Could you check a few things on this model? Use its own coordinates, in mm. Coordinates: 2 decimals unless noted, no trailing zeros. Write each loop counter-clockwise with the first axis right and the second up, starting at its lowest first coordinate (ties: lowest second). Pieces come first, ordered by that corner, then holes. Notation, with made-up numbers: M 69.5,-13 L 86.5,-13 A12 cw 86.5,-9 Z; hole C 76.25,68 d8. An arc over 180 degrees is marked long. Write item = value, one per line.
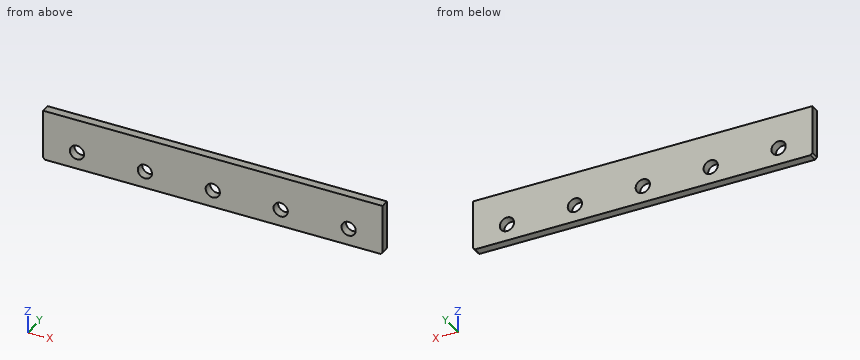
```python
from build123d import *

# Parameters (mm, degrees)
SKETCH1_W           = 127
SKETCH1_H           = 19.05
BOSS_EXTRUDE1_DEPTH = 3.175
SKETCH2_R           = 2.667
CUT_EXTRUDE1_DEPTH  = 3.175
CUT_EXTRUDE2_DEPTH  = 3.175


with BuildPart() as part:
    # Sketch1 → Boss-Extrude1 (new body)
    with BuildSketch(Plane(origin=(0, 0, 0), x_dir=(1, 0, 0), z_dir=(0, 1, 0))):
        Rectangle(SKETCH1_W, SKETCH1_H)
    extrude(amount=BOSS_EXTRUDE1_DEPTH)

    # Sketch2 → Cut-Extrude1 (cut)
    with BuildSketch(Plane(origin=(0, 3.175, 0), x_dir=(1, 0, 0), z_dir=(0, 1, 0))):
        with Locations((50.8, 3.175)):
            Circle(SKETCH2_R)
        with Locations((25.4, 3.175)):
            Circle(SKETCH2_R)
        with Locations((0, 3.175)):
            Circle(SKETCH2_R)
        with Locations((-25.4, 3.175)):
            Circle(SKETCH2_R)
        with Locations((-50.8, 3.175)):
            Circle(SKETCH2_R)
    extrude(amount=-CUT_EXTRUDE1_DEPTH, mode=Mode.SUBTRACT)

    # Sketch3 → Cut-Extrude2 (cut)
    with BuildSketch(Plane(origin=(0, 3.175, 0), x_dir=(1, 0, 0), z_dir=(0, 1, 0))):
        Polygon((-63.5, 9.525), (-63.5, 8.763), (-62.738, 9.525), align=None)
        Polygon((63.5, 9.525), (63.5, 8.763), (62.738, 9.525), align=None)
    extrude(amount=-CUT_EXTRUDE2_DEPTH, mode=Mode.SUBTRACT)


solid = part.part
```
Item 1: I'm going to push a flat-ended pin straight in: P1, Ø4.5, axis at x = -25.4, z = -3.175, coming from the -Y side. Where does the tip first touch, or does it pass through?
Numbers:
P1 = through
Item 2: Imagine slicing it at A-A (x = 25.4). Write out the boundary of the cut face in (y, z) (3 decimals), and give its area (3 significant figures).
Numbers:
outline = M 0,-9.525 L 3.175,-9.525 L 3.175,-5.842 L 0,-5.842 Z; M 0,-0.508 L 3.175,-0.508 L 3.175,9.525 L 0,9.525 Z
area = 43.5 mm²
Item 3: Imagine slicing it at B-B (y = 2.35). Write out the boundary of the cut face in (x, z) (3 decimals).
Numbers:
outline = M -63.5,-8.763 L -62.738,-9.525 L 62.738,-9.525 L 63.5,-8.763 L 63.5,9.525 L -63.5,9.525 Z; hole C -50.8,-3.175 d5.334; hole C -25.4,-3.175 d5.334; hole C 0,-3.175 d5.334; hole C 25.4,-3.175 d5.334; hole C 50.8,-3.175 d5.334
Item 4: If I drill on line 1 along Z through (x, y) = (0, 2.5) (3 decimals); line 2 along X through (y, z) = (2.75, -0.75); line 3 along X through (y, z) = (2.5, -1), over which ranges is the centre line in solid material (lowest first)?
Numbers:
line_1 = -9.525 to -5.842, -0.508 to 9.525
line_2 = -63.5 to -51.91, -49.69 to -26.51, -24.29 to -1.11, 1.11 to 24.29, 26.51 to 49.69, 51.91 to 63.5
line_3 = -63.5 to -52.34, -49.26 to -26.94, -23.86 to -1.54, 1.54 to 23.86, 26.94 to 49.26, 52.34 to 63.5
